Check sheet for the modelled part. Datum: model origin and axes. Units: mm. A direction names the side the tool comes from. Give positions to 0.01 mm unless a question says otherwise; leave off trailing zeros. Order: outer loops, then holes, each group sorted by start corner. A loop starts at its lowest first (then second) coordinate and runs counter-clockwise, first axis right, second up. Notation, with made-up numbers: (-17.75, 68.5) -> (18.25, 68.5) arc R17 cw to (18.25, 94.5) -> close; hole circle Ø1 at (35.5, 28.5). An arc over 180 degrees is marked (long way). One line per question, with ' | ' between items.
```python
from build123d import *

# Parameters (mm, degrees)
SKETCH1_W           = 15
SKETCH1_H           = 60
BOSS_EXTRUDE1_DEPTH = 103
SKETCH2_W           = 15
SKETCH2_H           = 2
BOSS_EXTRUDE2_DEPTH = 15
SKETCH3_W           = 15
SKETCH3_H           = 2
BOSS_EXTRUDE3_DEPTH = 15
SKETCH4_R           = 2.15
CUT_EXTRUDE1_DEPTH  = 15
CHAMFER2_SIZE       = 1


with BuildPart() as part:
    # Sketch1 → Boss-Extrude1 (new body)
    with BuildSketch(Plane(origin=(0, 0, 0), x_dir=(1, 0, 0), z_dir=(0, 1, 0))):
        with Locations((7.5, 30)):
            Rectangle(SKETCH1_W, SKETCH1_H)
    extrude(amount=BOSS_EXTRUDE1_DEPTH)

    # Sketch2 → Boss-Extrude2 (add)
    with BuildSketch(Plane(origin=(15, 0, 0), x_dir=(0, 0, -1), z_dir=(1, 0, 0))):
        with Locations((30, 1)):
            Rectangle(SKETCH2_W, SKETCH2_H)
    extrude(amount=BOSS_EXTRUDE2_DEPTH)

    # Sketch3 → Boss-Extrude3 (add)
    with BuildSketch(Plane.ZY):
        with Locations((-30, 1)):
            Rectangle(SKETCH3_W, SKETCH3_H)
    extrude(amount=BOSS_EXTRUDE3_DEPTH)

    # Sketch4 → Cut-Extrude1 (cut)
    with BuildSketch(Plane(origin=(0, 2, 0), x_dir=(1, 0, 0), z_dir=(0, 1, 0))):
        with Locations(Location((22.5, 30, 0), (0, 0, 270))):
            Circle(SKETCH4_R)
        with Locations(Location((-7.5, 30, 0), (0, 0, 270))):
            Circle(SKETCH4_R)
    extrude(amount=-CUT_EXTRUDE1_DEPTH, mode=Mode.SUBTRACT)

    # Chamfer2
    chamfer2_edges = [part.edges().sort_by_distance(p)[0] for p in [
        (22.5, 2, -32.15),
        (-7.5, 2, -32.15),
    ]]
    chamfer(chamfer2_edges, length=CHAMFER2_SIZE)


solid = part.part
```
Q1. Depth check by flat-ended pin: pin 1 Ø1 at (y, z) = (83.5, -22) entering from +X; pin 2 Ø18 at (y, z) = (32, -38.5) entering from -X; pin 3 Ø4.5 at (x, z) = (-9.5, -30) entering from +Y; pin 4 Ø3.5 at (x, z) = (22.5, -30) entering from +Y. Enter the tip coordinate at first touch or a pass-through.
Result sheet:
pin 1: stops at x = 15 | pin 2: stops at x = 0 | pin 3: stops at y = 2 | pin 4: passes through
Q2. Section check C-C (y = 69). Enter the section's corners in (x, z), and give its area (3 significant figures).
Result sheet:
outline: (0, -60) -> (15, -60) -> (15, 0) -> (0, 0) -> close | area: 900 mm2
Q3. Access from +Z, -Z, +X, -X, +Y, -Y to the whole of each face (thin tool, end or side, straight path). Record for faces 4 (the face through (22, 1, -37.5)), 5 (the face through (-7, 1, -37.5)), 6 (the face through (-7, 1, -22.5)), 7 (the face through (-7.4, 2, -33.4)).
Result sheet:
face 4: -Z, +X, +Y, -Y | face 5: -Z, -X, +Y, -Y | face 6: +Z, -X, +Y, -Y | face 7: +Z, -Z, -X, +Y
Q4. Section check D-D (z = -40). Enter the section's corners in (x, y).
Result sheet:
outline: (0, 0) -> (15, 0) -> (15, 103) -> (0, 103) -> close
Q5. Thickness scan on line 1 (X direction, y = 0.6, z = -30); line 2 (X direction, y = 11.5, z = -47); line 3 (Y direction, x = 21, z = -35). Record the ranges inside material, lowest first.
Result sheet:
line 1: x = -15 to -9.65, -5.35 to 20.35, 24.65 to 30 | line 2: x = 0 to 15 | line 3: y = 0 to 2
Q6. Section check A-A (x = 22.5). Enter the section's corners in (y, z), and give its area (3 significant figures).
Result sheet:
outline: (0, -37.5) -> (2, -37.5) -> (2, -33.15) -> (1, -32.15) -> (0, -32.15) -> close; (0, -27.85) -> (1, -27.85) -> (2, -26.85) -> (2, -22.5) -> (0, -22.5) -> close | area: 20.4 mm2
Q7. Mould release check, pull along Z, two halves, no side actions. Record for faces 1 (the face through (20.59, 0.51, -29.01)), 2 (the face through (19, 2, -30)), 3 (the face through (7, 51, -60)): pulls with the +Z half, pulls with the -Z half, needs draft (parallel to the pull), parting line crosses it, or undercut.
Result sheet:
face 1: undercut | face 2: needs draft | face 3: pulls with the -Z half
Q8. Section check B-B (z = -30). Enter the section's corners in (x, y), and give its area (3 significant figures).
Result sheet:
outline: (-15, 0) -> (-9.65, 0) -> (-9.65, 1) -> (-10.65, 2) -> (-15, 2) -> close; (-5.35, 0) -> (20.35, 0) -> (20.35, 1) -> (19.35, 2) -> (15, 2) -> (15, 103) -> (0, 103) -> (0, 2) -> (-4.35, 2) -> (-5.35, 1) -> close; (24.65, 0) -> (30, 0) -> (30, 2) -> (25.65, 2) -> (24.65, 1) -> close | area: 1,590 mm2
